```python
from build123d import *

# Parameters (mm, degrees)
CROQUIS1_W              = 250
CROQUIS1_H              = 150
SALIENTE_EXTRUIR1_DEPTH = 20
REDONDEO1_R             = 10
VACIADO2_T              = -2
SALIENTE_EXTRUIR2_START = 40
CROQUIS2_R              = 2.5
CROQUIS2_R_2            = 1
SALIENTE_EXTRUIR2_DEPTH = 40
SALIENTE_EXTRUIR3_START = -40
CROQUIS2_3_R            = 2.5
CROQUIS2_3_R_2          = 1
SALIENTE_EXTRUIR3_DEPTH = 40


with BuildPart() as part:
    # Croquis1 → Saliente-Extruir1 (new, symmetric)
    with BuildSketch(Plane(origin=(0, 0, 0), x_dir=(1, 0, 0), z_dir=(0, 1, 0))):
        Rectangle(CROQUIS1_W, CROQUIS1_H)
    extrude(amount=SALIENTE_EXTRUIR1_DEPTH, both=True)

    # Redondeo1
    redondeo1_edges = [part.edges().sort_by_distance(p)[0] for p in [
        (-125, -20, 0),
        (0, -20, -75),
        (125, -20, 0),
        (0, -20, 75),
        (-125, 0, 75),
        (-125, 0, -75),
        (125, 0, -75),
        (125, 0, 75),
    ]]
    fillet(redondeo1_edges, radius=REDONDEO1_R)

    # Vaciado2
    vaciado2_openings = [part.faces().sort_by_distance(p)[0] for p in [
        (0, 20, 0),
    ]]
    offset(amount=VACIADO2_T, openings=vaciado2_openings, kind=Kind.INTERSECTION)

    # Croquis2 → Saliente-Extruir2 (add)
    # profile 1 of 2: a face of its own
    with BuildSketch(Plane(origin=(0, 0, 0), x_dir=(0, 0, -1), z_dir=(1, 0, 0)).offset(SALIENTE_EXTRUIR2_START)):
        with BuildLine():
            Line((75, 11), (80.079542319, 18.612374783))
            ThreePointArc((80.079542319, 18.612374783), (77.275036483, 17.607422332), (75.5, 20))
            Line((75.5, 20), (75, 19))
            Line((75, 19), (75, 11))
        make_face()
    # profile 2 of 2: a face of its own
    with BuildSketch(Plane(origin=(0, 0, 0), x_dir=(0, 0, -1), z_dir=(1, 0, 0)).offset(SALIENTE_EXTRUIR2_START)):
        with Locations((78, 20)):
            Circle(CROQUIS2_R)
        with Locations((78, 20)):
            Circle(CROQUIS2_R_2, mode=Mode.SUBTRACT)
    extrude(amount=SALIENTE_EXTRUIR2_DEPTH)

    # Croquis2_3 → Saliente-Extruir3 (add)
    # profile 1 of 2: a face of its own
    with BuildSketch(Plane(origin=(0, 0, 0), x_dir=(0, 0, -1), z_dir=(1, 0, 0)).offset(SALIENTE_EXTRUIR3_START)):
        with BuildLine():
            Line((75, 11), (80.079542319, 18.612374783))
            ThreePointArc((80.079542319, 18.612374783), (77.275036483, 17.607422332), (75.5, 20))
            Line((75.5, 20), (75, 19))
            Line((75, 19), (75, 11))
        make_face()
    # profile 2 of 2: a face of its own
    with BuildSketch(Plane(origin=(0, 0, 0), x_dir=(0, 0, -1), z_dir=(1, 0, 0)).offset(SALIENTE_EXTRUIR3_START)):
        with Locations((78, 20)):
            Circle(CROQUIS2_3_R)
        with Locations((78, 20)):
            Circle(CROQUIS2_3_R_2, mode=Mode.SUBTRACT)
    extrude(amount=SALIENTE_EXTRUIR3_DEPTH)


solid = part.part
```
Work out the finished part from the listing and answer in its coordinate system (mm). A direction names the side the tool comes from. Round coordinates to 2 decimals unless told otherwise and drop trailing zeros. Loops run counter-clockwise (first coordinate to the right, second up) from the corner with the lowest first, then second, coordinate; pieces in that order, holes last. Notation, with made-up numbers: (-5.75, 74) -> (26.25, 74) arc R22 ccw to (26.25, 81) -> close; hole circle Ø6 at (21.5, 52). An arc over 180 degrees is marked (long way). Write each question's results on one line, items separated by ' | '. Start each with the question number.
1. Find the intervals of material crossed by probe 1 along X at (y, z) = (18, -34); probe 2 along Z at (x, y) = (107, 15); probe 3 along Y at (x, z) = (48, 28), in increasing order. Write a range as from..to.
2. Section C-C (z = 3) is taken. Determine the outline of the cut face in (x, y).
3. Section D-D (x = -100) is taken. Determine the outline of the cut face in (y, z).
4. Section A-A (x = -20) is taken. Determine the outline of the cut face in (y, z), plus the area to 3 significant figures.
5. A tool of negligible diameter and unlimited length cuts with its end or side. For faces 1 (the face through (-123, 5, 1)), 2 (the face through (-122.15, 5.21, 71.99)), from which of +Z, -Z, +X, -X, +Y, -Y can it reach the whole face along a straight path? Write none if from no direction.
6. For a pull along X with two mould halves and no side action, classify faces 3 (the face through (-20.28, 22.37, -78.79)), 4 (the face through (0, 18, -77)), 5 (the face through (-40, 18, -77)), 6 (the face through (80, 18, -77)) as +X half, -X half, draft (parallel to the pull), parting line (faces both ways), or undercut.
7. Section B-B (y = -4.5) is taken. Determine the outline of the cut face in (x, z).
8. Given pin 1 Ø6 at (y, z) = (19.5, -78.5) entering from -X; pin 2 Ø5 at (x, z) = (74.5, -48.5) entering from +Y; pin 3 Ø15 at (x, y) = (-10, 2.5) entering from -Z; pin 4 Ø2 at (y, z) = (-11, 29.5) entering from -X, each flat-ended and moving along its own axis, determine where each tip first touches the part or whether it passes through.
Evaluation:
1) probe 1: x = -125..-123, 123..125 | probe 2: z = -75..-73, 73..75 | probe 3: y = -20..-18
2) outline: (-125, -10) arc R10 ccw to (-115, -20) -> (115, -20) arc R10 ccw to (125, -10) -> (125, 20) -> (123, 20) -> (123, -10) arc R8 cw to (115, -18) -> (-115, -18) arc R8 cw to (-123, -10) -> (-123, 20) -> (-125, 20) -> close
3) outline: (-20, -65) arc R10 ccw to (-10, -75) -> (20, -75) -> (20, -73) -> (-10, -73) arc R8 cw to (-18, -65) -> (-18, 65) arc R8 cw to (-10, 73) -> (20, 73) -> (20, 75) -> (-10, 75) arc R10 ccw to (-20, 65) -> close
4) outline: (-20, -65) arc R10 ccw to (-10, -75) -> (11, -75) -> (18.61, -80.08) arc R2.5 ccw (long way) to (20, -75.5) -> (19, -75) -> (20, -75) -> (20, -73) -> (-10, -73) arc R8 cw to (-18, -65) -> (-18, 65) arc R8 cw to (-10, 73) -> (20, 73) -> (20, 75) -> (-10, 75) arc R10 ccw to (-20, 65) -> close; hole circle Ø2 at (20, -78) | area: 470 mm2
5) face 1: +Y | face 2: +Z, -X, +Y, -Y
6) face 3: draft | face 4: undercut | face 5: -X half | face 6: +X half
7) outline: (-125, -65) arc R10 ccw to (-115, -75) -> (115, -75) arc R10 ccw to (125, -65) -> (125, 65) arc R10 ccw to (115, 75) -> (-115, 75) arc R10 ccw to (-125, 65) -> close; hole (-123, -65) arc R8 ccw to (-115, -73) -> (115, -73) arc R8 ccw to (123, -65) -> (123, 65) arc R8 ccw to (115, 73) -> (-115, 73) arc R8 ccw to (-123, 65) -> close
8) pin 1: stops at x = -40 | pin 2: stops at y = -18 | pin 3: stops at z = -75 | pin 4: stops at x = -125
